```python
from build123d import *

# Parameters (mm, degrees)
SKETCH1_W           = 38.675
SKETCH1_H           = 5
SKETCH3_R           = 4.1
SKETCH3_R_2         = 2.3
CUT_EXTRUDE4_DEPTH  = 55.92277533
CHAMFER1_SIZE       = 0.5
CUT_EXTRUDE11_DEPTH = 3
CHAMFER2_SIZE       = 0.5
CHAMFER3_SIZE       = 0.25


with BuildPart() as part:
    # Sketch1 → Revolve1 (revolve)
    with BuildSketch(Plane(origin=(0, 0, 0), x_dir=(1, 0, 0), z_dir=(0, 1, 0)), mode=Mode.PRIVATE) as revolve1_sk:
        with Locations((-19.3375, 2.5)):
            Rectangle(SKETCH1_W, SKETCH1_H)
    revolve(revolve1_sk.sketch.rotate(Axis((0, 0, 0), (0, 0, -1)), 180), axis=Axis((0, 0, 0), (0, 0, -1)))

    # Sketch3 → Cut-Extrude4 (cut, through all)
    with BuildSketch(Plane(origin=(0, 0, 0), x_dir=(-1, 0, 0), z_dir=(0, 0, -1))):
        Circle(SKETCH3_R)
        with Locations((-12.5, 21.650635095)):
            Circle(SKETCH3_R_2)
        with Locations((12.5, 21.650635095)):
            Circle(SKETCH3_R_2)
        with Locations((25, 0)):
            Circle(SKETCH3_R_2)
        with Locations((12.5, -21.650635095)):
            Circle(SKETCH3_R_2)
        with Locations((-12.5, -21.650635095)):
            Circle(SKETCH3_R_2)
        with Locations((-25, 0)):
            Circle(SKETCH3_R_2)
    extrude(amount=CUT_EXTRUDE4_DEPTH, mode=Mode.SUBTRACT)

    # Chamfer1
    chamfer1_edges = [part.edges().sort_by_distance(p)[0] for p in [
        (-38.675, 0, 0),
        (-38.675, 0, -5),
    ]]
    chamfer(chamfer1_edges, length=CHAMFER1_SIZE)

    # Sketch14 → Cut-Extrude11 (cut)
    with BuildSketch(Plane.XY):
        with BuildLine():
            Line((-2.871572225, 26.543373742), (-5.522750274, 17.77635457))
            ThreePointArc((-5.522750274, 17.77635457), (-6.564563598, 15.785168894), (-8.265894724, 14.316949631))
            ThreePointArc((-8.265894724, 14.316949631), (-10.388075466, 13.577663288), (-12.633399507, 13.67101932))
            Line((-12.633399507, 13.67101932), (-21.55144985, 15.758541367))
            ThreePointArc((-21.55144985, 15.758541367), (-24.833278454, 14.3375), (-24.423022075, 10.784832375))
            Line((-24.423022075, 10.784832375), (-18.156149781, 4.105335249))
            ThreePointArc((-18.156149781, 4.105335249), (-16.952639064, 2.207505606), (-16.531789447, 0))
            ThreePointArc((-16.531789447, 0), (-16.952639064, -2.207505606), (-18.156149781, -4.105335249))
            Line((-18.156149781, -4.105335249), (-24.423022075, -10.784832375))
            ThreePointArc((-24.423022075, -10.784832375), (-24.833278454, -14.3375), (-21.55144985, -15.758541367))
            Line((-21.55144985, -15.758541367), (-12.633399507, -13.67101932))
            ThreePointArc((-12.633399507, -13.67101932), (-10.388075466, -13.577663288), (-8.265894724, -14.316949631))
            ThreePointArc((-8.265894724, -14.316949631), (-6.564563598, -15.785168894), (-5.522750274, -17.77635457))
            Line((-5.522750274, -17.77635457), (-2.871572225, -26.543373742))
            ThreePointArc((-2.871572225, -26.543373742), (0, -28.675), (2.871572225, -26.543373742))
            Line((2.871572225, -26.543373742), (5.522750274, -17.77635457))
            ThreePointArc((5.522750274, -17.77635457), (6.564563598, -15.785168894), (8.265894724, -14.316949631))
            ThreePointArc((8.265894724, -14.316949631), (10.388075466, -13.577663288), (12.633399507, -13.67101932))
            Line((12.633399507, -13.67101932), (21.55144985, -15.758541367))
            ThreePointArc((21.55144985, -15.758541367), (24.833278454, -14.3375), (24.423022075, -10.784832375))
            Line((24.423022075, -10.784832375), (18.156149781, -4.105335249))
            ThreePointArc((18.156149781, -4.105335249), (16.952639064, -2.207505606), (16.531789447, 0))
            ThreePointArc((16.531789447, 0), (16.952639064, 2.207505606), (18.156149781, 4.105335249))
            Line((18.156149781, 4.105335249), (24.423022075, 10.784832375))
            ThreePointArc((24.423022075, 10.784832375), (24.833278454, 14.3375), (21.55144985, 15.758541367))
            Line((21.55144985, 15.758541367), (12.633399507, 13.67101932))
            ThreePointArc((12.633399507, 13.67101932), (10.388075466, 13.577663288), (8.265894724, 14.316949631))
            ThreePointArc((8.265894724, 14.316949631), (6.564563598, 15.785168894), (5.522750274, 17.77635457))
            Line((5.522750274, 17.77635457), (2.871572225, 26.543373742))
            ThreePointArc((2.871572225, 26.543373742), (0, 28.675), (-2.871572225, 26.543373742))
        make_face()
    extrude(amount=-CUT_EXTRUDE11_DEPTH, mode=Mode.SUBTRACT)

    # Chamfer2
    chamfer2_edges = [part.edges().sort_by_distance(p)[0] for p in [
        (0, 28.675, -3),
        (4.197161249, 22.159864156, -3),
        (8.265894724, 14.316949631, -3),
        (17.092424679, 14.714780344, -3),
        (24.833278454, 14.3375, -3),
        (21.289585928, 7.445083812, -3),
        (16.531789447, 0, -3),
        (21.289585928, -7.445083812, -3),
        (24.833278454, -14.3375, -3),
        (17.092424679, -14.714780344, -3),
        (8.265894724, -14.316949631, -3),
        (4.197161249, -22.159864156, -3),
        (0, -28.675, -3),
        (-4.197161249, -22.159864156, -3),
        (-8.265894724, -14.316949631, -3),
        (-17.092424679, -14.714780344, -3),
        (-24.833278454, -14.3375, -3),
        (-21.289585928, -7.445083812, -3),
        (-16.531789447, 0, -3),
        (-21.289585928, 7.445083812, -3),
        (-24.833278454, 14.3375, -3),
        (-17.092424679, 14.714780344, -3),
        (-8.265894724, 14.316949631, -3),
        (-4.197161249, 22.159864156, -3),
        (0, 28.675, 0),
        (-4.197161249, 22.159864156, 0),
        (-8.265894724, 14.316949631, 0),
        (-17.092424679, 14.714780344, 0),
        (-24.833278454, 14.3375, 0),
        (-21.289585928, 7.445083812, 0),
        (-16.531789447, 0, 0),
        (-21.289585928, -7.445083812, 0),
        (-24.833278454, -14.3375, 0),
        (-17.092424679, -14.714780344, 0),
        (-8.265894724, -14.316949631, 0),
        (-4.197161249, -22.159864156, 0),
        (0, -28.675, 0),
        (4.197161249, -22.159864156, 0),
        (8.265894724, -14.316949631, 0),
        (17.092424679, -14.714780344, 0),
        (24.833278454, -14.3375, 0),
        (21.289585928, -7.445083812, 0),
        (16.531789447, 0, 0),
        (21.289585928, 7.445083812, 0),
        (24.833278454, 14.3375, 0),
        (17.092424679, 14.714780344, 0),
        (8.265894724, 14.316949631, 0),
        (4.197161249, 22.159864156, 0),
    ]]
    chamfer(chamfer2_edges, length=CHAMFER2_SIZE)

    # Chamfer3
    chamfer3_edges = [part.edges().sort_by_distance(p)[0] for p in [
        (14.8, 21.650635095, 0),
        (14.8, 21.650635095, -5),
        (-10.2, 21.650635095, 0),
        (-10.2, 21.650635095, -5),
        (-22.7, 0, 0),
        (-22.7, 0, -5),
        (-10.2, -21.650635095, 0),
        (-10.2, -21.650635095, -5),
        (14.8, -21.650635095, 0),
        (14.8, -21.650635095, -5),
        (27.3, 0, 0),
        (27.3, 0, -5),
        (4.1, 0, -5),
        (4.1, 0, -3),
    ]]
    chamfer(chamfer3_edges, length=CHAMFER3_SIZE)


solid = part.part
```
Source: CAD feature listing. Evaluate the final solid. Frame: model axes, mm. A direction names the side the tool comes from. Give positions to 0.01 mm unless a question says otherwise; leave off trailing zeros. Loops run counter-clockwise (first coordinate to the right, second up) from the corner with the lowest first, then second, coordinate; pieces in that order, holes last. Notation, with made-up numbers: M 58,-11 L 115,-11 A16 cw 115,19 Z; hole C 89,-32 d7. An arc over 180 degrees is marked long. Put each result on its own line as item: value.
Q1. Section A-A (x = 0). Return the cut outline in (y, z) (3 decimals).
Response values:
outline: M -38.675,-4.5 L -38.175,-5 L -4.35,-5 L -4.1,-4.75 L -4.1,-3.25 L -4.35,-3 L -28.175,-3 L -28.675,-2.5 L -28.675,-0.5 L -29.175,0 L -38.175,0 L -38.675,-0.5 Z; M 4.1,-4.75 L 4.35,-5 L 38.175,-5 L 38.675,-4.5 L 38.675,-0.5 L 38.175,0 L 29.175,0 L 28.675,-0.5 L 28.675,-2.5 L 28.175,-3 L 4.35,-3 L 4.1,-3.25 Z
Q2. Section B-B (z = -1.7). Count the separate pieces of the cut face and the enclosed holes in it, and give its area (3 significant figures).
Response values:
separate pieces: 1
enclosed holes: 7
area: 3,120 mm²
Q3. Reachability of faces 1 (the flat face through (21.513, -7.323, -0.253)), 2 (the cylindrical face through (14.798, -21.55, -2.468)) from +Z, -Z, +X, -X, +Y, -Y: full face, straight path, thin tool, end or side. Return the list, or none.
Response values:
face 1: +Z
face 2: +Z, -Z
Q4. Line query: probe 1 along Y at (x, z) = (12.5, -2.2); probe 2 along X at (y, z) = (-30, -4.4); probe 3 along Z at (x, y) = (-16, -6.5). Output: solid intervals per line, ascending. Write a range as [from, to].
Response values:
probe 1: y = [-36.6, -23.95], [-19.35, -13.64], [13.64, 19.35], [23.95, 36.6]
probe 2: x = [-24.41, 24.41]
probe 3: z = [-5, -3]
Q5. Pin query (flat end, axial travel): P1, Ø3, axis at x = -9, y = 2, coming from the +Z side. Return the tip coordinate at first contact, or that it passes through.
Response values:
P1: stops at z = -3
